```python
from build123d import *

# Parameters (mm, degrees)
SKETCH1_R           = 38.1
BOSS_EXTRUDE1_DEPTH = 101.6
SKETCH3_R           = 34.29
CUT_EXTRUDE2_DEPTH  = 101.6
SKETCH4_R           = 1.27
BOSS_EXTRUDE2_DEPTH = 6.35
CUT_EXTRUDE5_DEPTH  = 95.25


with BuildPart() as part:
    # Sketch1 → Boss-Extrude1 (new body)
    with BuildSketch(Plane(origin=(0, 0, 0), x_dir=(1, 0, 0), z_dir=(0, 1, 0))):
        with Locations(Location((0, 0, 0), (0, 0, 270))):
            Circle(SKETCH1_R)
    extrude(amount=BOSS_EXTRUDE1_DEPTH)

    # Sketch2 → Revolve1 (revolve)
    with BuildSketch(Plane(origin=(0, 0, 0), x_dir=(0, 0, -1), z_dir=(1, 0, 0))):
        with BuildLine():
            Line((38.1, 101.6), (34.29, 101.6))
            ThreePointArc((34.29, 101.6), (24.246691527, 125.846691527), (0, 135.89))
            Line((0, 135.89), (0, 139.7))
            ThreePointArc((0, 139.7), (26.940768363, 128.540768363), (38.1, 101.6))
        make_face()
    revolve(axis=Axis((0, 0, 0), (0, 1, 0)))

    # Sketch3 → Cut-Extrude2 (cut)
    with BuildSketch(Plane.XZ):
        with Locations(Location((0, 0, 0), (0, 0, 270))):
            Circle(SKETCH3_R)
    extrude(amount=-CUT_EXTRUDE2_DEPTH, mode=Mode.SUBTRACT)

    # Sketch4 → Boss-Extrude2 (add)
    with BuildSketch(Plane(origin=(0, 0, 0), x_dir=(1, 0, 0), z_dir=(0, 1, 0))):
        with Locations(Location((0, -35.56, 0), (0, 0, 270))):
            Circle(SKETCH4_R)
        with Locations(Location((-30.795863359, -17.78, 0), (0, 0, 270))):
            Circle(SKETCH4_R)
        with Locations(Location((-30.795863359, 17.78, 0), (0, 0, 270))):
            Circle(SKETCH4_R)
        with Locations(Location((0, 35.56, 0), (0, 0, 270))):
            Circle(SKETCH4_R)
        with Locations(Location((30.795863359, 17.78, 0), (0, 0, 270))):
            Circle(SKETCH4_R)
        with Locations(Location((30.795863359, -17.78, 0), (0, 0, 270))):
            Circle(SKETCH4_R)
    extrude(amount=-BOSS_EXTRUDE2_DEPTH)

    # Sketch5 → Cut-Extrude5 (cut)
    with BuildSketch(Plane.XZ):
        Polygon((-21.563277102, 32.196696757), (-17.195234057, 34.790265717), (-14.171362758, 29.697515071), (-18.539405803, 27.103946111), align=None)
        Polygon((14.203002973, 29.607569452), (18.633121102, 27.12151769), (21.531636887, 32.286642376), (17.101518758, 34.772694138), align=None)
        Polygon((32.742408776, 2.503623341), (32.804483859, -2.575997381), (38.726870944, -2.503623341), (38.66479586, 2.575997381), align=None)
        Polygon((18.539405803, -27.103946111), (14.171362758, -29.697515071), (17.195234057, -34.790265717), (21.563277102, -32.196696757), align=None)
        Polygon((-14.203002973, -29.607569452), (-18.633121102, -27.12151769), (-21.531636887, -32.286642376), (-17.101518758, -34.772694138), align=None)
        Polygon((-32.742408776, -2.503623341), (-32.804483859, 2.575997381), (-38.726870944, 2.503623341), (-38.66479586, -2.575997381), align=None)
    extrude(amount=-CUT_EXTRUDE5_DEPTH, mode=Mode.SUBTRACT)


solid = part.part
```
The model under review builds one solid part; all positions refer to its coordinate system, in mm. A direction names the side the tool comes from. Give positions to 0.01 mm unless a question says otherwise; leave off trailing zeros. Loops run counter-clockwise (first coordinate to the right, second up) from the corner with the lowest first, then second, coordinate; pieces in that order, holes last. Notation, with made-up numbers: (-29.75, -33) - (-21.75, -33) arc R29 cw to (-21.75, -4) - close; hole circle Ø1 at (81.25, 80). An arc over 180 degrees is marked (long way). Answer as a JSON object with one key per item and string values.
Q1. Add section D-D on y = 99. State the section outline as (x, z) points, plus the area to 3 significant figures.
Worked out:
{"outline": "circle Ø76.2 at (0, 0); hole circle Ø68.58 at (0, 0)", "area": "866 mm^2"}
Q2. To check wall thickness, follow line 1 along Z through (x, y) = (0, 79); line 2 along X through (y, z) = (125.5, -21.5); line 3 along X through (y, z) = (100, 12). State the ranges of each line that lie inside material, in increasing order.
Worked out:
{"line 1": "z = -38.1 to -34.29, 34.29 to 38.1", "line 2": "x = -20.45 to -11.93, 11.93 to 20.45", "line 3": "x = -36.16 to -32.12, 32.12 to 36.16"}
Q3. Add section C-C on x = -5. State the section outline as (y, z) points, plus the area to 3 significant figures.
Worked out:
{"outline": "(0, -37.77) - (101.6, -37.77) arc R37.77 ccw to (101.6, 37.77) - (0, 37.77) - (0, 33.92) - (101.6, 33.92) arc R33.92 cw to (101.6, -33.92) - (0, -33.92) - close", "area": "1,210 mm^2"}
Q4. Add section A-A on y = 78. State the section outline as (x, z) points, plus the area to 3 significant figures.
Worked out:
{"outline": "(-38.02, 2.51) - (-34.19, 2.56) arc R34.29 cw to (-19.28, 28.35) - (-21.23, 31.64) arc R38.1 ccw to start; (-38.01, -2.57) arc R38.1 ccw to (-21.18, -31.67) - (-19.31, -28.33) arc R34.29 cw to (-34.2, -2.52) - close; (-16.83, 34.18) - (-14.88, 30.89) arc R34.29 cw to (14.91, 30.88) - (16.78, 34.2) arc R38.1 ccw to start; (-16.78, -34.2) arc R38.1 ccw to (16.83, -34.18) - (14.88, -30.89) arc R34.29 cw to (-14.91, -30.88) - close; (19.28, -28.35) - (21.23, -31.64) arc R38.1 ccw to (38.02, -2.51) - (34.19, -2.56) arc R34.29 cw to start; (19.31, 28.33) arc R34.29 cw to (34.2, 2.52) - (38.01, 2.57) arc R38.1 ccw to (21.18, 31.67) - close", "area": "750 mm^2"}
Q5. Mouldability with a two-part tool opening along X and no side actions: class faces 4 (the flat face through (0, 0, 37)), 5 (the flat face through (-20.24, 46.96, 29.97)), 6 (the cylindrical face through (-23.183, 50.089, -30.235)) as +X half, -X half, draft (parallel to the pull), parting line (faces both ways), or undercut.
Worked out:
{"face 4": "draft", "face 5": "undercut", "face 6": "parting line"}
Q6. Add section B-B on z = 0. State the section outline as (x, y) points.
Worked out:
{"outline": "(-38.1, 95.25) - (-34.29, 95.25) - (-34.29, 101.6) arc R34.29 cw to (34.29, 101.6) - (34.29, 95.25) - (38.1, 95.25) - (38.1, 101.6) arc R38.1 ccw to (-38.1, 101.6) - close"}
Q7. For faces 1 (the flat face through (-18, 95.25, -31)), 2 (the flat face through (20.27, 46.96, -30.02)), 3 (the flat face through (20.236, 46.958, 29.977)), list the 3-axis set-ups (+Z, -Z, +X, -X, +Y, -Y) from which the entire face can be reached by the end or side of a thin tool; tool diameter is ignored.
Worked out:
{"face 1": "-Y", "face 2": "-Z, -Y", "face 3": "+Z, -Y"}
Q8. Insertion check: pin 1 (4 mm diameter, centred on x = -3.5, y = 100, fed in from -Z); pin 2 (3 mm diameter, centred on x = -12.5, y = 54.5, fed in from +Z); pin 3 (1.5 mm diameter, centred on y = 63, z = -21, fed in from -X). Each pin has a flat end and moves straight along its axis. Give the tip position at first contact, or say it passes through.
Worked out:
{"pin 1": "stops at z = -38.07", "pin 2": "stops at z = 36.48", "pin 3": "stops at x = -32.27"}
